Here's how the part is built. I have some questions about the finished solid (model axes, mm). A direction names the side the tool comes from. Round coordinates to 2 decimals unless told otherwise and drop trailing zeros. Loops run counter-clockwise (first coordinate to the right, second up) from the corner with the lowest first, then second, coordinate; pieces in that order, holes last. Notation, with made-up numbers: M 61.25,7 L 66.25,7 A28 ccw 66.25,34 Z; hole C 58.25,-5.5 d1. An arc over 180 degrees is marked long. Answer as a JSON object with one key per item and string values.
from build123d import *

# Parameters (mm, degrees)
BOSS_EXTRU_4_DEPTH = 140
BOSS_EXTRU_5_REACH = 142.319
ESQUISSE2_W        = 14.6
ESQUISSE2_H        = 5
ESQUISSE4_W        = 14.6
ESQUISSE4_H        = 5
BOSS_EXTRU_6_DEPTH = 10


with BuildPart() as part:
    # Esquisse1 → Boss.-Extru.4 (new body)
    with BuildSketch(Plane.XY):
        Polygon((-7.3, 0), (-7.3, -6), (-4.3, -6), (-4.3, -2), (4.3, -2), (4.3, -6), (7.3, -6), (7.3, 0), align=None)
    extrude(amount=BOSS_EXTRU_4_DEPTH)

    # Esquisse2 → Boss.-Extru.5 (add, up to next)
    with BuildSketch(Plane.XZ.offset(6), mode=Mode.PRIVATE) as boss_extru_5_sk1:
        with Locations((0, 2.5)):
            Rectangle(ESQUISSE2_W, ESQUISSE2_H)
    boss_extru_5_tool1 = extrude(boss_extru_5_sk1.sketch, amount=-BOSS_EXTRU_5_REACH, mode=Mode.PRIVATE) - part.part
    add(boss_extru_5_tool1.solids().sort_by_distance((0, -6, 2.5))[0])

    # Esquisse4 → Boss.-Extru.6 (add)
    with BuildSketch(Plane(origin=(0, 0, 0), x_dir=(1, 0, 0), z_dir=(0, 1, 0))):
        with Locations((0, -137.5)):
            Rectangle(ESQUISSE4_W, ESQUISSE4_H)
    extrude(amount=-BOSS_EXTRU_6_DEPTH)


solid = part.part
Item 1: I want a section at A-A, the plane x = 3. Please give me the cut outline in (y, z), then the cut area to 3 significant figures.
Resolved:
{"outline": "M -10,135 L -2,135 L -2,5 L -6,5 L -6,0 L 0,0 L 0,140 L -10,140 Z", "area": "340 mm²"}
Item 2: I'm going to push flat-ended pins straight in: pin 1 Ø2 at (x, z) = (-2, 44.5) entering from +Y; pin 2 Ø7 at (x, z) = (2, 42.5) entering from -Y; pin 3 Ø4.5 at (x, z) = (2, 44.5) entering from -Y. Where does each tip first touch, or does it pass through?
Resolved:
{"pin 1": "y = 0", "pin 2": "y = -6", "pin 3": "y = -2"}
Item 3: I want a section at C-C, the plane z = 23.5. Please give me the cut outline in (x, y), then the cut area to 3 significant figures.
Resolved:
{"outline": "M -7.3,-6 L -4.3,-6 L -4.3,-2 L 4.3,-2 L 4.3,-6 L 7.3,-6 L 7.3,0 L -7.3,0 Z", "area": "53.2 mm²"}
Item 4: If we mould it in two halves opening along Z, with no side actions, what happens to faces 1 (the face through (7.3, -3, 69)), 2 (the face through (0, -3, 0)), 3 (the face through (4.3, -4, 69))? For each: pulls with the +Z half, pulls with the -Z half, needs draft (parallel to the pull), parting line crosses it, or undercut.
Resolved:
{"face 1": "needs draft", "face 2": "pulls with the -Z half", "face 3": "undercut"}
Item 5: Please list where these lines run through material, in increasing order: probe 1 along X at (y, z) = (-2.25, 104); probe 2 along Z at (x, y) = (-3.5, -4.25); probe 3 along Z at (x, y) = (6.75, -7.5). Write a range as from..to.
Resolved:
{"probe 1": "-7.3..-4.3, 4.3..7.3", "probe 2": "0..5, 135..140", "probe 3": "135..140"}
Item 6: On a 3-axis mill with a long thin cutter (end or side, diameter ignored), from which of +Z, -Z, +X, -X, +Y, -Y can I reach the whole of each face in a straight line? I mean faces 4 (the face through (-5, -6, 68)), 5 (the face through (0, -5, 140)), 6 (the face through (0, -2, 69)). Say none if no direction works.
Resolved:
{"face 4": "-Z, +X, -X, -Y", "face 5": "+Z, +X, -X, +Y, -Y", "face 6": "-Y"}
Item 7: I want a section at B-B, the plane y = -3.5. Please give me the cut outline in (x, z).
Resolved:
{"outline": "M -7.3,0 L 7.3,0 L 7.3,140 L -7.3,140 Z; hole M -4.3,5 L 4.3,5 L 4.3,135 L -4.3,135 Z"}
